Input: part model. Units: mm. Frame: model coordinates. A direction names the side the tool comes from. Round coordinates to 2 decimals unless told otherwise and drop trailing zeros. Loops run counter-clockwise (first coordinate to the right, second up) from the corner with the lowest first, then second, coordinate; pieces in that order, holes last. Notation, with made-up numbers: M 39.5,60.5 L 53.5,60.5 A8 ccw 53.5,68.5 Z; hole C -20,51.5 d5. An arc over 180 degrees is marked long. Use one line per item in the form item = value. Start each with the question number.
Q1. Ray query, line 1 along X through (y, z) = (42, 2.75); line 2 along X through (y, z) = (-19, 9); line 3 along X through (y, z) = (18, 5.25). Return the intervals inside material, ascending.
Q2. Section query C-C, the plane y = 49.5. Output: boundary loops of the cut face in (x, z).
Q3. Mould query, pull axis X, two halves, no side actions, for faces 3 (the cylindrical face through (70.17, -20.33, 6.26)), 4 (the flat face through (30, -40.685, 6)), 5 (the cylindrical face through (-61.965, 33.269, 6.439)), 6 (the flat face through (-47.45, -17.87, 6.26)). Classes: pulls with the +X half, pulls with the -X half, needs draft (parallel to the pull), parting line crosses it, or undercut.
Q4. Section query A-A, the plane x = 15. Output: boundary loops of the cut face in (y, z), and give its area (3 significant figures).
Q5. Access query for faces 1 (the flat face through (40.081, 51, 6)), 2 (the flat face through (-11, 33, 12.7)). Directions: +Z, -Z, +X, -X, +Y, -Y. A direction counts if a zero-diameter tool reaches every point of the face in a straight line with its end or side. Return the directions, or none.
Q6. First-contact query: P1, Ø6.5, axis at y = 56, z = 3.5, coming from the +X side; P2, Ø4, axis at x = 52, z = 5.5, coming from the +Y side. Flat tips, straight axial feed; report the tip coordinate or a pass-through.
Q7. Section query B-B, the plane z = 10.25. State how many separate pieces and enclosed holes the cut face has, and give its area (3 significant figures).
Q8. Section query D-D, the plane x = 56. Output: boundary loops of the cut face in (y, z).
Autodesk Inventor part; units mm, degrees
ref_plane "YZ Plane" through (0, 0, 0) normal (1, 0, 0) x (0, 1, 0)
ref_plane "XZ Plane" through (0, 0, 0) normal (0, 1, 0) x (-1, 0, 0)
ref_plane "XY Plane" through (0, 0, 0) normal (0, 0, 1) x (1, 0, 0)
sketch "Esboço1" plane through (0, 0, 0) normal (0, 0, 1) x (1, 0, 0)
  line L0 (-70.9188, 104.3152) -> (40.0812, 104.3152)
  line L1 (-70.9188, 5.5999) -> (-70.9188, 104.3152)
  line L2 (-24.6341, -40.6848) -> (86.1475, -40.6848)
  line L3 (86.1475, -40.6848) -> (86.1475, -0.6848)
  line L4 (86.1475, -0.6848) -> (40.0812, -0.6848)
  line L5 (40.0812, -0.6848) -> (40.0812, 104.3152)
  line L6 (-24.6341, -40.6848) -> (-70.9188, 5.5999)
  line L7 (-24.6341, -40.6848) -> (40.8222, -40.6848) construction
  point P0 (0, 0)
  dimension "d0" = 111
  dimension "d5" = 40
  dimension "d6" = 105
  dimension "d7" = 135
  dimension "d8" = 98.7154
  dimension "d11" = 157.0662
extrude "Extrusão1" add sketch "Esboço1" along normal blind 12.7
chamfer "Chanfro1" distance 20 angle 45 1 edges at (-70.9188, 104.3152, 6.35)
sketch "Esboço2" plane through (0, 0, 0) normal (0, 0, -1) x (-1, 0, 0)
  circle A0 centre (45.7988, 78.3152) radius 2.75 construction
  circle A1 centre (63.7988, 78.3152) radius 2.75 construction
  circle A2 centre (63.7988, 32.3152) radius 2.75 construction
  circle A3 centre (45.7988, 32.3152) radius 2.75 construction
  point P0 (0, 0)
hole "Furo1" at (-45.7988, 78.3152, 0) at (-63.7988, 78.3152, 0) at (-45.7988, 32.3152, 0) at (-63.7988, 32.3152, 0) direction (0, 0, 1) diameter 4.134 end through all
sketch "Esboço3" plane through (0, 0, 12.7) normal (0, 0, 1) x (1, 0, 0)
  circle A0 centre (12.5812, -20.6848) radius 4.25 construction
  circle A1 centre (12.5812, 19.3152) radius 4.25 construction
  line L0 (40.0812, -0.6848) -> (40.0812, 104.3152)
  line L1 (-24.6341, -40.6848) -> (86.1475, -40.6848)
  point P0 (0, 0)
  dimension "d22" = 27.5
  dimension "d23" = 27.5
  dimension "d24" = 60
  dimension "d25" = 20
hole "Furo2" at (12.5812, 19.3152, 12.7) at (12.5812, -20.6848, 12.7) direction (0, 0, -1) diameter 8.5 end through all
sketch "Esboço4" plane through (0, 0, 12.7) normal (0, 0, 1) x (1, 0, 0)
  circle A0 centre (46.3975, -20.6848) radius 2.75 construction
  circle A1 centre (72.8975, -20.6848) radius 2.75 construction
  line L0 (86.1475, -40.6848) -> (86.1475, -0.6848)
  line L1 (86.1475, -0.6848) -> (40.0812, -0.6848)
  line L2 (-24.6341, -40.6848) -> (86.1475, -40.6848)
  point P0 (0, 0)
  dimension "d33" = 13.25
  dimension "d34" = 39.75
  dimension "d35" = 20
  dimension "d36" = 20
hole "Furo3" at (46.3975, -20.6848, 12.7) at (72.8975, -20.6848, 12.7) direction (0, 0, -1) diameter 5.5 end through all
properties part number "SUPORTE_MANCAL_FRONTAL"
Results found:
q1.line_1 = -70.92 to 40.08
q1.line_2 = -46.32 to 8.68, 16.48 to 44.22, 48.57 to 70.72, 75.07 to 86.15
q1.line_3 = -70.92 to 8.54, 16.62 to 40.08
q2.outline = M -70.92,0 L 40.08,0 L 40.08,12.7 L -70.92,12.7 Z
q3.face_3 = undercut
q3.face_4 = needs draft
q3.face_5 = undercut
q3.face_6 = pulls with the -X half
q4.outline = M -40.68,0 L -24.18,0 L -24.18,12.7 L -40.68,12.7 Z; M -17.19,0 L 15.82,0 L 15.82,12.7 L -17.19,12.7 Z; M 22.81,0 L 104.32,0 L 104.32,12.7 L 22.81,12.7 Z
q4.area = 1,660 mm²
q5.face_1 = +Z, -Z, +X, +Y
q5.face_2 = +Z, +X, -X, +Y, -Y
q6.P1 = 40.08
q6.P2 = -0.68
q7.separate_pieces = 1
q7.enclosed_holes = 8
q7.area = 16,500 mm²
q8.outline = M -40.68,0 L -0.68,0 L -0.68,12.7 L -40.68,12.7 Z
